Part model, mm, in its own coordinate system. Give positions to 0.01 mm unless a question says otherwise; leave off trailing zeros. Loops run counter-clockwise (first coordinate to the right, second up) from the corner with the lowest first, then second, coordinate; pieces in that order, holes last. Notation, with made-up numbers: M 39.5,25.5 L 58.5,25.5 A20 ccw 58.5,51.5 Z; hole C 56.5,-4 d9. An arc over 180 degrees is marked long. Put each result on its own line as item: value. Start each with the question number.
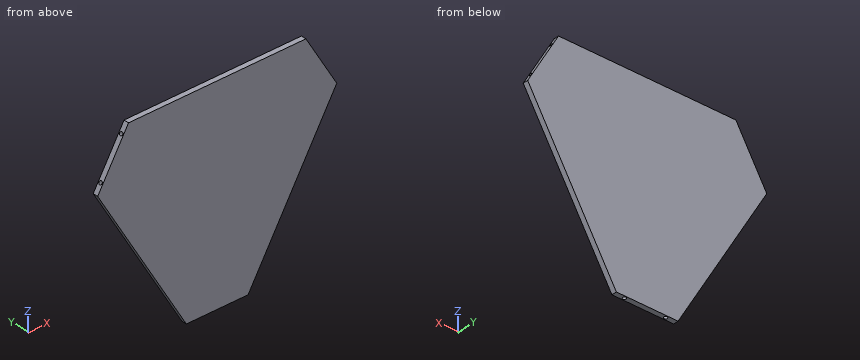
```python
from build123d import *

# Parameters (mm, degrees)
BOSS_EXTRUDE1_DEPTH            = 6.35
M5X0_8_TAPPED_HOLE1_AT_2_COUNT = 2
M5X0_8_TAPPED_HOLE1_AT_2_PITCH = 50.8
CIRPATTERN1_COUNT              = 3


with BuildPart() as part:
    # Sketch1 → Boss-Extrude1 (new body)
    with BuildSketch(Plane(origin=(0, 0, 0), x_dir=(1, 0, 0), z_dir=(0, 1, 0))):
        Polygon((-147.591032992, -41.217632116), (-109.491032992, -107.208767884), (109.491032992, -107.208767884), (147.591032992, -41.217632116), (38.1, 148.4264), (-38.1, 148.4264), align=None)
    extrude(amount=BOSS_EXTRUDE1_DEPTH)

    # Sketch3 → M5x0.8 Tapped Hole1 (revolve, cut)
    with BuildSketch(Plane(origin=(115.841032992, 3.175, 96.210245256), x_dir=(0.5, 0, -0.866025404), z_dir=(0, 1, 0))):
        Polygon((0, 0), (0, 13.9618073), (2.1, 12.7), (2.1, 0), align=None)
    m5x0_8_tapped_hole1 = revolve(axis=Axis((121.340294306, 3.175, 99.385245256), (-0.866025404, 0, -0.5)), mode=Mode.SUBTRACT)

    # M5x0.8 Tapped Hole1 at 2: M5x0.8 Tapped Hole1 ×2
    with Locations(*[Vector(0.5, 0, -0.866025404) * (i * M5X0_8_TAPPED_HOLE1_AT_2_PITCH) for i in range(1, M5X0_8_TAPPED_HOLE1_AT_2_COUNT)]):
        add(m5x0_8_tapped_hole1, mode=Mode.SUBTRACT)

    # CirPattern1: M5x0.8 Tapped Hole1 ×3 about axis
    cirpattern1_axis = Axis((0, 6.6675, 0), (0, -1, 0))
    for i in range(1, CIRPATTERN1_COUNT):
        add(m5x0_8_tapped_hole1.rotate(cirpattern1_axis, i * 360 / CIRPATTERN1_COUNT), mode=Mode.SUBTRACT)

    # CirPattern1 copy 1 sketch → CirPattern1 copy 1 (revolve, cut)
    with BuildSketch(Plane(origin=(-115.841032992, 3.175, 96.210245256), x_dir=(0.5, 0, 0.866025404), z_dir=(0, 1, 0))):
        Polygon((0, 0), (0, 13.9618073), (2.1, 12.7), (2.1, 0), align=None)
    revolve(axis=Axis((-121.340294306, 3.175, 99.385245256), (0.866025404, 0, -0.5)), mode=Mode.SUBTRACT)

    # CirPattern1 copy 2 sketch → CirPattern1 copy 2 (revolve, cut)
    with BuildSketch(Plane(origin=(-25.4, 3.175, -148.4264), x_dir=(-1, 0, 0), z_dir=(0, 1, 0))):
        Polygon((0, 0), (0, 13.9618073), (2.1, 12.7), (2.1, 0), align=None)
    revolve(axis=Axis((-25.4, 3.175, -154.7764), (0, 0, 1)), mode=Mode.SUBTRACT)


solid = part.part
```
1) Pin check, flat tips, straight feed: pin 1 Ø3 at (x, y) = (56, 4.5) entering from -Z; pin 2 Ø1 at (x, y) = (-116.5, 4) entering from -Z. Stop position of each tip, or through.
2) Band-saw the part on A-A on z = -109. Give the cut face in (x, y).
3) Wall check: L1, parallel to Y at x = -25.4, z = -140.25 (3 decimals); L2, parallel to Z at x = -126.5, y = 5.5; L3, parallel to X at y = 1.5, z = -37. Give the ranges that are in metal, low to high.
4) Band-saw the part on B-B on x = 94. Give the cut face in (y, z).
Evaluation:
1. pin 1: z = -120.02
1. pin 2: z = -13.5
2. outline: M -60.86,0 L 60.86,0 L 60.86,6.35 L -60.86,6.35 Z
3. L1: 0 to 1.075, 5.275 to 6.35
3. L2: 4.69 to 77.75
3. L3: -102.43 to 102.43
4. outline: M 0,-51.6 L 6.35,-51.6 L 6.35,107.21 L 0,107.21 Z
